```python
from build123d import *

# Parameters (mm, degrees)
F1_DEPTH = 15


with BuildPart() as f1:
    # F0 (on Front) → F1 (new body)
    with BuildSketch(Plane.XZ):
        Polygon((0, 42.300776), (0, 54.800776), (-54.800776, 0), (-42.300776, 0), align=None)
        Polygon((-42.300776, 0), (-54.800776, 0), (-60, 0), (-60, -10.1), (0, -10.1), (0, 0), align=None)
    extrude(amount=F1_DEPTH)


solid = f1.part
```
Geometry: final body of the model. Coordinates: model frame, mm. A direction names the side the tool comes from. Give positions to 0.01 mm unless a question says otherwise; leave off trailing zeros. Loops run counter-clockwise (first coordinate to the right, second up) from the corner with the lowest first, then second, coordinate; pieces in that order, holes last. Notation, with made-up numbers: (-3, 4.5) - (13, 4.5) arc R20 ccw to (13, 10.5) - close; hole circle Ø10 at (51, -26). An arc over 180 degrees is marked (long way). Answer as CSV lines item,"result". Start each with the question number.
(1) Section query D-D (z = 21). Output: boundary loops of the cut face in (x, y), and give its area (4 significant figures).
(2) Pin query (flat end, axial travel): P1, Ø1.6, axis at x = -56, y = -8, coming from the +Z side; P2, Ø5, axis at y = -8, z = 15.5, coming from the -X side; P3, Ø1.5, axis at y = -10.5, z = 38.5, coming from the -X side; P4, Ø3, axis at x = -40.5, z = 17, coming from the +Y side. Return the tip coordinate at first contact, or that it passes through.
(3) Section query C-C (x = -47). Output: boundary loops of the cut face in (y, z).
(4) Mould query, pull axis Z, two halves, no side actions, for faces 3 (the face through (-30, 0, 13)), 4 (the face through (-21, -7, 0)), 5 (the face through (-30, -7, -10.1)), 6 (the face through (-57, -7, 0)). Classes: +Z half, -Z half, draft (parallel to the pull), parting line (faces both ways), or undercut.
(5) Ray query, line 1 along Z through (x, y) = (-15, -9.25); line 2 along Z through (x, y) = (-58, -7.5); line 3 along Z through (x, y) = (-37, -12). Return the intervals inside material, ascending. Write a range as [from, to].
(6) Section query B-B (y = -1). Output: boundary loops of the cut face in (x, z), and give its area (3 significant figures).
(7) Section query A-A (x = -10). Output: boundary loops of the cut face in (y, z).
(8) Reachability of faces 1 (the face through (-21.4, -7.4, 20.9)), 2 (the face through (0, -7, 48)) from +Z, -Z, +X, -X, +Y, -Y: full face, straight path, thin tool, end or side. Return the list, or none.
Worked answers:
1,outline,"(-33.8, -15) - (-21.3, -15) - (-21.3, 0) - (-33.8, 0) - close"
1,area,"187.5 mm^2"
2,P1,"stops at z = 0"
2,P2,"stops at x = -41.8"
2,P3,"stops at x = -17.05"
2,P4,"passes through"
3,outline,"(-15, -10.1) - (0, -10.1) - (0, 7.8) - (-15, 7.8) - close"
4,face 3,"draft"
4,face 4,"undercut"
4,face 5,"-Z half"
4,face 6,"+Z half"
5,line 1,"z = [-10.1, 0], [27.3, 39.8]"
5,line 2,"z = [-10.1, 0]"
5,line 3,"z = [-10.1, 0], [5.3, 17.8]"
6,outline,"(-60, -10.1) - (0, -10.1) - (0, 0) - (-42.3, 0) - (0, 42.3) - (0, 54.8) - (-54.8, 0) - (-60, 0) - close"
6,area,"1,210 mm^2"
7,outline,"(-15, -10.1) - (0, -10.1) - (0, 0) - (-15, 0) - close; (-15, 32.3) - (0, 32.3) - (0, 44.8) - (-15, 44.8) - close"
8,face 1,"+X, +Y, -Y"
8,face 2,"+Z, -Z, +X, +Y, -Y"
